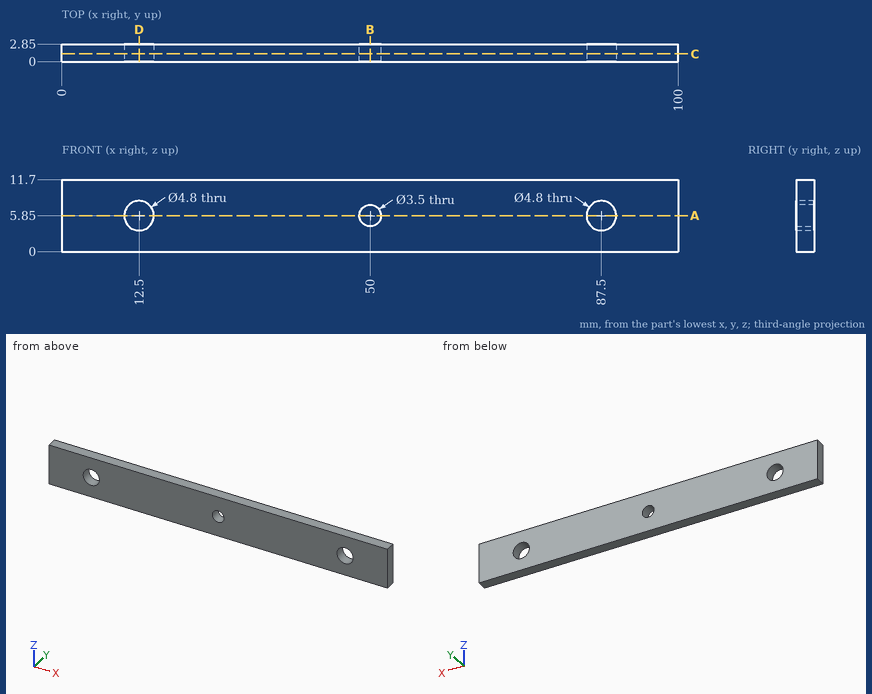
Study the drawing (mm; zero at the part's minimum x, y, z) and answer. Round coordinates to 2 decimals unless told otherwise and drop trailing zeros. Write each loop counter-clockwise with the first axis right and the second up, starting at its lowest first coordinate (ties: lowest second). Pieces come first, ordered by that corner, then holes. Notation, with made-up numbers: (15, 66.25) -> (73, 66.25) arc R13 ccw to (73, 90.25) -> close; hole circle Ø5 at (16, 64). An arc over 180 degrees is marked (long way). Use CSV: the item, a comma, the result in double quotes. Start each with the question number.
(1) Consider L1, parallel to X at y = 0.6, z = 5.85; L2, parallel to X at y = 0.2, z = 5.25; L3, parallel to Z at x = 14.5, y = 1.6. Determine where each line is inside the solid, lowest interval first. Write a range as from..to.
(2) Section A-A on z = 5.85 is taken. Give the vertices of the cut face in (x, y), then the cut area to 3 significant figures.
(3) This flat-tipped pin is pushed along its axis until it touches: pin 1 (3 mm diameter, centred on x = 50, z = 5.85, fed in from +Y). Where does it stop, or does it pass through?
(4) Section B-B on x = 50 is taken. Give the vertices of the cut face in (y, z).
(5) Section D-D on x = 12.5 is taken. Give the vertices of the cut face in (y, z).
(6) Section C-C on y = 1.25 is taken. Give the vertices of the cut face in (x, z).
A:
1,L1,"x = 0..10.1, 14.9..48.25, 51.75..85.1, 89.9..100"
1,L2,"x = 0..10.18, 14.82..48.36, 51.64..85.18, 89.82..100"
1,L3,"z = 0..4.52, 7.18..11.7"
2,outline,"(0, 0) -> (10.1, 0) -> (10.1, 2.85) -> (0, 2.85) -> close; (14.9, 0) -> (48.25, 0) -> (48.25, 2.85) -> (14.9, 2.85) -> close; (51.75, 0) -> (85.1, 0) -> (85.1, 2.85) -> (51.75, 2.85) -> close; (89.9, 0) -> (100, 0) -> (100, 2.85) -> (89.9, 2.85) -> close"
2,area,"248 mm²"
3,pin 1,"passes through"
4,outline,"(0, 0) -> (2.85, 0) -> (2.85, 4.1) -> (0, 4.1) -> close; (0, 7.6) -> (2.85, 7.6) -> (2.85, 11.7) -> (0, 11.7) -> close"
5,outline,"(0, 0) -> (2.85, 0) -> (2.85, 3.45) -> (0, 3.45) -> close; (0, 8.25) -> (2.85, 8.25) -> (2.85, 11.7) -> (0, 11.7) -> close"
6,outline,"(0, 0) -> (100, 0) -> (100, 11.7) -> (0, 11.7) -> close; hole circle Ø4.8 at (12.5, 5.85); hole circle Ø3.5 at (50, 5.85); hole circle Ø4.8 at (87.5, 5.85)"
